Autodesk Inventor part; units mm, degrees
ref_plane "YZ Plane" through (0, 0, 0) normal (1, 0, 0) x (0, 1, 0)
ref_plane "XZ Plane" through (0, 0, 0) normal (0, 1, 0) x (-1, 0, 0)
ref_plane "XY Plane" through (0, 0, 0) normal (0, 0, 1) x (1, 0, 0)
sketch "Эскиз1" plane through (0, 0, 0) normal (0, 1, 0) x (-1, 0, 0)
  line L0 (-5, -19) -> (5, -19)
  line L1 (5, -19) -> (5, 19)
  line L2 (5, 19) -> (-5, 19)
  line L3 (-5, 19) -> (-5, -19)
  line L4 (-5, -19) -> (5, 19) construction
  line L5 (5, -19) -> (-5, 19) construction
  line L6 (5, 0) -> (5, 12)
  line L7 (5, 12) -> (45, 12)
  line L8 (45, 12) -> (45, 0)
  line L9 (30, 0) -> (5, 0)
  line L10 (45, 0) -> (45, 4)
  line L11 (45, 4) -> (30, 4)
  line L12 (30, 4) -> (30, 0)
  line L13 (45, 12) -> (45, 11)
  line L14 (45, 11) -> (29, 11)
  line L15 (29, 11) -> (29, 12)
  line L16 (45, 4) -> (30, 4)
  line L17 (30, 4) -> (30, -4)
  line L18 (30, -4) -> (45, -4)
  line L19 (45, -4) -> (45, 4)
  line L20 (29, -11) -> (29, -12)
  line L21 (29, -12) -> (45, -12)
  line L22 (45, -12) -> (45, -11)
  line L23 (45, -11) -> (29, -11)
  line L24 (29, -11) -> (29, -12)
  line L25 (5, 12) -> (8, 12)
  line L26 (5, 0) -> (5, 11.75)
  line L27 (5, 11.75) -> (8, 11.75)
  line L28 (8, 11.75) -> (8, 12)
  line L29 (5, 11.75) -> (6, 11.75)
  line L30 (6, 11.75) -> (6, 12.75)
  line L31 (6, 12.75) -> (5, 12.75)
  line L32 (5, 12.75) -> (5, 11.75)
  circle A0 centre (6, 12.75) radius 1
  line L33 (8, 12) -> (6, 11.75)
  point P0 (0, 0)
  point P1 (6.2462, 11.7808)
  dimension "d0" = 10
  dimension "d1" = 38
  dimension "d2" = 12
  dimension "d3" = 40
  dimension "d4" = 4
  dimension "d5" = 15
  dimension "d6" = 1
  dimension "d7" = 16
  dimension "d13" = 8
  dimension "d14" = 22
  dimension "d15" = 1
  dimension "d60" = 3
  dimension "d61" = 11.75
  dimension "d62" = 1
  dimension "d63" = 1
extrude "Выдавливание1" add sketch "Эскиз1" along normal mid plane 46 contours L3 L2 L1 L0
revolve "Вращение1" add sketch "Эскиз1" angle 360 about axis through (-30, 0, 0) along (1, 0, 0) contours L1 L27 L28 L7 L15 L14 L8 L11 L12 L9 | L1 L7 A0 L27 | A0 L7 L1 | A0 L33 L28 L27 | L14 L15 L7 L8
extrude "Выдавливание3" cut sketch "Эскиз1" along normal mid plane 46 contours L12 L11 L8 L19 L18 L17 | L14 L15 L7 L8 | L23 L22 L21 L20
sketch "Эскиз3" plane through (-29, 4.7958, -11) normal (0, 0, -1) x (-1, 0, 0)
  line L0 (16, -9.5917) -> (16, 0)
  circle A0 centre (16, -4.7958) radius 8.5
  point P0 (-29, -4.7958)
  dimension "d21" = 17
extrude "Выдавливание5" cut sketch "Эскиз3" against normal blind 39
sketch "Эскиз4" plane through (5, -23, -19) normal (1, 0, 0) x (0, 0, -1)
  line L0 (-19, 23) -> (-19, 39)
  line L1 (-19, 39) -> (-31, 39)
  line L2 (-19, 23) -> (-19, 7)
  line L3 (-19, 7) -> (-7, 7)
  line L4 (-19, 7) -> (-31, 7)
  line L5 (-19, 39) -> (-7, 39)
  dimension "d24" = 16
  dimension "d25" = 12
  dimension "d26" = 16
  dimension "d27" = 12
  dimension "d28" = 12
hole "Отверстие3" at (5, 16, -12) at (5, -16, 12) direction (-1, 0, 0) diameter 7 end through all counterbore diameter 12 counterbore depth 7
hole "Отверстие4" at (5, -16, -12) direction (-1, 0, 0) diameter 8 end through all
chamfer "Фаска1" distance 2 angle 45 4 edges at (0, 23, -19) (0, -23, -19) (0, -23, 19) (0, 23, 19)
properties part number "Фиксатор-11"
Input: part model. Units: mm. Frame: model coordinates. A direction names the side the tool comes from. Give positions to 0.01 mm unless a question says otherwise; leave off trailing zeros. Order: outer loops, then holes, each group sorted by start corner. A loop starts at its lowest first (then second) coordinate and runs counter-clockwise, first axis right, second up.
Q1. Section C-C on y = -16. Output: boundary loops of the cut face in (x, z), and give its area (3 significant figures).
Checked values:
outline: (-5, -19) - (5, -19) - (5, -16) - (-5, -16) - close; (-5, -8) - (5, -8) - (5, 6) - (-2, 6) - (-2, 8.5) - (-5, 8.5) - close; (-5, 15.5) - (-2, 15.5) - (-2, 18) - (5, 18) - (5, 19) - (-5, 19) - close
area: 195 mm2
Q2. Contact query for flat-ended pins moving along their axis: pin 1 Ø3.5 at (y, z) = (-17.5, 10) entering from +X; pin 2 Ø4.5 at (x, y) = (-32, -2) entering from -Z; pin 3 Ø8 at (y, z) = (15.5, 12) entering from -X; pin 4 Ø5.5 at (y, z) = (16, -12) entering from +X. Output: stop coordinate, or through.
Checked values:
pin 1: stops at x = -2
pin 2: stops at z = -11
pin 3: stops at x = -5
pin 4: passes through
Q3. Section D-D on z = 0. Output: boundary loops of the cut face in (x, y).
Checked values:
outline: (-30, -12) - (-8, -12) - (-6.25, -11.78) arc R1 cw to (-5, -12.75) - (-5, -23) - (5, -23) - (5, 23) - (-5, 23) - (-5, 12.75) arc R1 cw to (-6.25, 11.78) - (-8, 12) - (-30, 12) - close
Q4. Section A-A on x = -4. Output: boundary loops of the cut face in (y, z), and give its area (3 significant figures).
Checked values:
outline: (-23, -17) - (-21, -19) - (21, -19) - (23, -17) - (23, 17) - (21, 19) - (-21, 19) - (-23, 17) - close; hole circle Ø8 at (-16, -12); hole circle Ø7 at (-16, 12); hole circle Ø7 at (16, -12)
area: 1,610 mm2
Q5. Draft query along Z for faces 6 (the flat face through (0, -22, 18)), 7 (the flat face through (0, 22, -18)), 8 (the cylindrical face through (-3.52, -19.47, 12.46)). Return one class per face: +Z half, -Z half, draft (parallel to the pull), parting line (faces both ways), or undercut.
Checked values:
face 6: +Z half
face 7: -Z half
face 8: undercut
Q6. Section B-B on y = 16. Output: boundary loops of the cut face in (x, z).
Checked values:
outline: (-5, -19) - (5, -19) - (5, -18) - (-2, -18) - (-2, -15.5) - (-5, -15.5) - close; (-5, -8.5) - (-2, -8.5) - (-2, -6) - (5, -6) - (5, 19) - (-5, 19) - close
Q7. Set-up query: faces 1 (the cylindrical face through (1.451, -17.802, 6.277)), 2 (the flat face through (-34, 0, -11)), 3 (the cylindrical face through (-22.65, 0.53, -11.99)), 4 (the flat face through (-34, 0, 11)), 5 (the flat face through (-36, 0, -4)). Return all of +Z, -Z, +X, -X, +Y, -Y with unobstructed straight access to the full face (end or side cutting, diameter ignored); none if empty.
Checked values:
face 1: +X
face 2: -Z, -X, +Y, -Y
face 3: -X
face 4: +Z, -X, +Y, -Y
face 5: -X, +Y, -Y
Q8. Ray query, probe 1 along Z at (x, y) = (-3.8, -16); probe 2 along Y at (x, z) = (1, -12); probe 3 along Z at (x, y) = (2, 16). Return the intervals inside material, ascending.
Checked values:
probe 1: z = -19 to -16, -8 to 8.5, 15.5 to 19
probe 2: y = -23 to -20, -12 to 10, 22 to 23
probe 3: z = -19 to -18, -6 to 19
